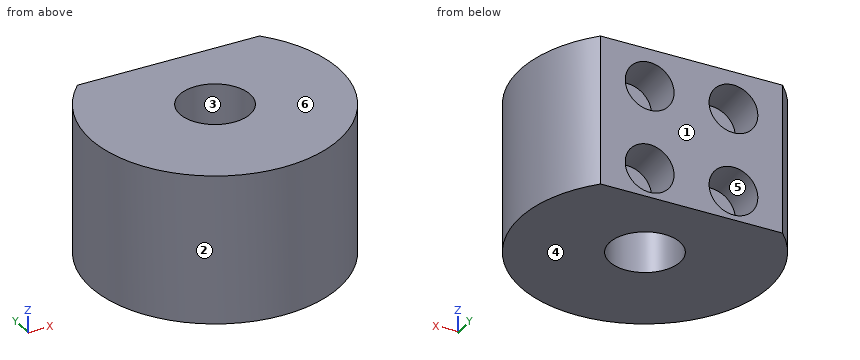
Solid Edge part; units mm, degrees
sketch "Sketch1" plane through (0, 0, 0) normal (0, 0, 1) x (1, 0, 0)
  circle A0 centre (0, 0) radius 15
  circle A1 centre (0, 0) radius 4.25
extrude "ExtrudedProtrusion_1" add sketch "Sketch1" against normal blind 18
sketch "Sketch2" plane through (0, 0, 0) normal (0, 0, 1) x (0, 1, 0)
  line L0 (10.35, -10.8571) -> (10.35, 10.8571)
  arc A0 (10.35, 10.8571) -> (10.35, -10.8571) centre (0, 0) cw
extrude "ExtrudedCutout_1" cut sketch "Sketch2" against normal blind 18
sketch "Sketch3" plane through (0, 10.35, -9) normal (0, 1, 0) x (-1, 0, 0)
  circle A0 centre (-5, 4.5) radius 2.9108
  circle A1 centre (5, 4.5) radius 2.9108
  circle A2 centre (-5, -5.5) radius 2.9108
  circle A3 centre (5, -5.5) radius 2.9108
extrude "ExtrudedCutout_2" cut sketch "Sketch3" against normal blind 5
properties material "ABS"
Read the model definition and answer for the solid it produces. Units are mm, in the model's axes. Face numbers are marked on the shaded views. A direction names the side the tool comes from. Round coordinates to 2 decimals unless told otherwise and drop trailing zeros. Order: outer loops, then holes, each group sorted by start corner. A loop starts at its lowest first (then second) coordinate and runs counter-clockwise, first axis right, second up. Notation, with made-up numbers: (31, 22) - (76, 22) arc R21 cw to (76, 27) - close; hole circle Ø8 at (39, -34.5). An arc over 180 degrees is marked (long way). Use one line per item in the form item = value. Start each with the question number.
(1) Determine the mould class of the marked faces 1, 2, 3 and 4 for opening direction Y: +Y half, -Y half, draft (parallel to the pull), parting line (faces both ways), or undercut.
(2) Find the intervals of material crossed by line 1 along Z through (x, y) = (-5, 7.35); line 2 along X through (y, z) = (8, -15.75); line 3 along X through (y, z) = (6.75, -12), in increasing order. Write a range as from..to.
(3) The part is cut by section C-C (x = 0). Give the vertices of the cut face in (y, z).
(4) The part is cut by section A-A (z = -14.5). Give the vertices of the cut face in (x, y).
(5) The part is cut by section B-B (y = 0). Give the vertices of the cut face in (x, z), then the cut area to 3 significant figures.
(6) Flat-ended cylindrical pins translate along their axes: pin 1 Ø9.5 at (x, z) = (5, -14.5) entering from -Y; pin 2 Ø8 at (y, z) = (-5.5, -14.5) entering from +X; pin 3 Ø3.5 at (x, z) = (-5, -14.5) entering from -Y. Find the tip coordinate at first contact, or state that the pin passes through.
(7) The part is cut by section D-D (x = -12). Give the vertices of the cut face in (y, z).
(8) For the marked faces 5 and 6, determine the directions among +Z, -Z, +X, -X, +Y, -Y from which every point of the face is accessible in a straight line to the end or side of a thin tool.
Checked values:
q1.face_1 = +Y half
q1.face_2 = parting line
q1.face_3 = undercut
q1.face_4 = draft
q2.line_1 = -18..-17.41, -11.59..-7.41, -1.59..0
q2.line_2 = -12.69..-7.63, -2.37..2.37, 7.63..12.69
q2.line_3 = -13.4..-6.49, -3.51..3.51, 6.49..13.4
q3.outline = (-15, -18) - (-4.25, -18) - (-4.25, 0) - (-15, 0) - close; (4.25, -18) - (10.35, -18) - (10.35, 0) - (4.25, 0) - close
q4.outline = (-10.86, 10.35) arc R15 ccw (long way) to (10.86, 10.35) - (7.91, 10.35) - (7.91, 5.35) - (2.09, 5.35) - (2.09, 10.35) - (-2.09, 10.35) - (-2.09, 5.35) - (-7.91, 5.35) - (-7.91, 10.35) - close; hole circle Ø8.5 at (0, 0)
q5.outline = (-15, -18) - (-4.25, -18) - (-4.25, 0) - (-15, 0) - close; (4.25, -18) - (15, -18) - (15, 0) - (4.25, 0) - close
q5.area = 387 mm^2
q6.pin_1 = -15
q6.pin_2 = 14.92
q6.pin_3 = -14.64
q7.outline = (-9, -18) - (9, -18) - (9, 0) - (-9, 0) - close
q8.face_5 = +Y
q8.face_6 = +Z, +X, -X, +Y, -Y
